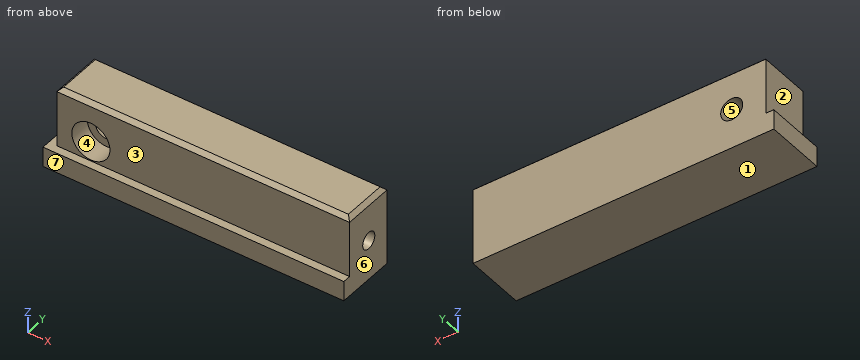
from build123d import *

# Parameters (mm, degrees)
F0_W           = 73
F0_H           = 20
F1_DEPTH       = 13
F2_W           = 75
F2_H           = 5
F3_DEPTH       = 2
F4_W           = 13
F4_H           = 5
F5_DEPTH       = 2
F7_D           = 5.5
F7_CBORE_D     = 9.5
F7_CBORE_DEPTH = 5.4
F9_D           = 4.2
F9_DEPTH       = 8
F9_TIP         = 1.2618073
F10_SIZE       = 1


with BuildPart() as f1:
    # F0 (on Front) → F1 (new body)
    with BuildSketch(Plane.XZ):
        with Locations((36.5, 10)):
            Rectangle(F0_W, F0_H)
    extrude(amount=F1_DEPTH)

    # F2 (on face) → F3 (join)
    with BuildSketch(Plane.XZ.offset(13)):
        with Locations((35.5, 2.5)):
            Rectangle(F2_W, F2_H)
    extrude(amount=F3_DEPTH)

    # F4 (on face) → F5 (join)
    with BuildSketch(Plane(origin=(0, 0, 0), x_dir=(0, -1, 0), z_dir=(-1, 0, 0))):
        with Locations((6.5, 2.5)):
            Rectangle(F4_W, F4_H)
    extrude(amount=F5_DEPTH)

    # F7 (through all)
    with Locations(Plane.XZ.offset(13)):
        with Locations((8.5, 10)):
            CounterBoreHole(F7_D / 2, F7_CBORE_D / 2, F7_CBORE_DEPTH)

    # F9
    with Locations(Plane.YZ.offset(73)):
        with Locations((-6.3317259774, 10)):
            Hole(F9_D / 2, depth=F9_DEPTH)
            with Locations((0, 0, -(F9_DEPTH + F9_TIP / 2))):  # 118° drill point
                Cone(0, F9_D / 2, F9_TIP, mode=Mode.SUBTRACT)

    # F10
    f10_edges = [f1.edges().sort_by_distance(p)[0] for p in [
        (36.5, 0, 20),
        (36.5, -13, 20),
        (0, -6.5, 20),
        (73, -6.5, 20),
    ]]
    chamfer(f10_edges, length=F10_SIZE)


solid = f1.part
Build history of the part. All positions in model axes, mm. Face numbers are marked on the shaded views. A direction names the side the tool comes from. Give positions to 0.01 mm unless a question says otherwise; leave off trailing zeros. Order: outer loops, then holes, each group sorted by start corner. A loop starts at its lowest first (then second) coordinate and runs counter-clockwise, first axis right, second up. Notation, with made-up numbers: M 9,61.5 L 62,61.5 A28 ccw 62,83.5 Z; hole C 57.25,-3.5 d9. An arc over 180 degrees is marked long. Use one line per item in the form item = value.
1) Probe probe 1 along Z at (x, y) = (8.5, -5.5); probe 2 along Z at (x, y) = (8.5, -8.95); probe 3 along X at (y, z) = (-11.5, 9.75). List the from-to ranges inside material, lowest first.
Calculated:
probe_1 = 0 to 7.25, 12.75 to 20
probe_2 = 0 to 5.25, 14.75 to 20
probe_3 = 0 to 3.76, 13.24 to 73
2) Saw through at A-A (x = 43). Give the cut face in (y, z).
Calculated:
outline = M -15,0 L 0,0 L 0,19 L -1,20 L -12,20 L -13,19 L -13,5 L -15,5 Z
3) Tool access for the marked faces 1, 2 and 3: list every direction of +Z, -Z, +X, -X, +Y, -Y with a clear straight run to the whole face (end or side of a thin tool).
Calculated:
face_1 = -Z, +X, -X, +Y, -Y
face_2 = +Z, -X, +Y, -Y
face_3 = +Z, +X, -X, -Y
4) Saw through at C-C (z = 15.5). Give the cut face in (x, y), plus the area to 3 significant figures.
Calculated:
outline = M 0,-13 L 73,-13 L 73,0 L 0,0 Z
area = 949 mm2
5) Two-plate mould, pull along X, no slides. Class the marked faces 4, 5, 6 and 7: released by +X, released by -X, zero draft, split by the parting line, or undercut.
Calculated:
face_4 = undercut
face_5 = undercut
face_6 = released by +X
face_7 = zero draft
6) Saw through at B-B (x = 8.5). Give the cut face in (y, z), plus the area to 3 significant figures.
Calculated:
outline = M -15,0 L 0,0 L 0,7.25 L -7.6,7.25 L -7.6,5.25 L -13,5.25 L -13,5 L -15,5 Z; M -13,14.75 L -7.6,14.75 L -7.6,12.75 L 0,12.75 L 0,19 L -1,20 L -12,20 L -13,19 Z
area = 176 mm2
7) Drop flat-ended pins along their axis: pin 1 (4 mm diameter, centred on y = -6.5, z = 14.5, fed in from -X); pin 2 (4 mm diameter, centred on x = 34, z = 9.5, fed in from -Y); pin 3 (3 mm diameter, centred on x = 9.5, z = 9, fed in from -Y). Give the stop position or say it passes through.
Calculated:
pin_1 = 0
pin_2 = -13
pin_3 = -7.6
